```python
from build123d import *

# Parameters (mm, degrees)
CROQUIS1_R              = 2.6
CROQUIS1_R_2            = 3.5
CROQUIS1_R_3            = 1.75
CROQUIS1_R_4            = 11.25
CROQUIS1_R_5            = 2.5
CROQUIS1_W              = 7.5
CROQUIS1_H              = 3
SALIENTE_EXTRUIR1_DEPTH = 6


with BuildPart() as part:
    # Croquis1 → Saliente-Extruir1 (new body)
    with BuildSketch(Plane.XY):
        Polygon((-50, -104.5), (-50, 45.5), (-41, 54.5), (-41, 84.5), (-50, 89.696152423), (-50, 104.5), (50, 104.5), (50, 89.696152423), (41, 84.5), (41, 54.5), (50, 45.5), (50, -104.5), (27, -104.5), (21, -98.5), (-21, -98.5), (-27, -104.5), align=None)
        with Locations((-35, -94.5)):
            Circle(CROQUIS1_R, mode=Mode.SUBTRACT)
        with Locations((-35, -34.5)):
            Circle(CROQUIS1_R_2, mode=Mode.SUBTRACT)
        with Locations((35, -34.5)):
            Circle(CROQUIS1_R_2, mode=Mode.SUBTRACT)
        with Locations((35, -94.5)):
            Circle(CROQUIS1_R, mode=Mode.SUBTRACT)
        with Locations((-15.5, 13.5)):
            Circle(CROQUIS1_R_3, mode=Mode.SUBTRACT)
        with Locations((15.5, 13.5)):
            Circle(CROQUIS1_R_3, mode=Mode.SUBTRACT)
        with Locations((0, 29)):
            Circle(CROQUIS1_R_4, mode=Mode.SUBTRACT)
        with Locations((15.5, 44.5)):
            Circle(CROQUIS1_R_3, mode=Mode.SUBTRACT)
        with Locations((-15.5, 44.5)):
            Circle(CROQUIS1_R_3, mode=Mode.SUBTRACT)
        with Locations((0, 69.5)):
            Circle(CROQUIS1_R_5, mode=Mode.SUBTRACT)
        with Locations((0, 89.5)):
            Circle(CROQUIS1_R_5, mode=Mode.SUBTRACT)
        with Locations((0, 56)):
            Rectangle(CROQUIS1_W, CROQUIS1_H, mode=Mode.SUBTRACT)
        with Locations((0, 63)):
            Rectangle(CROQUIS1_W, CROQUIS1_H, mode=Mode.SUBTRACT)
    extrude(amount=SALIENTE_EXTRUIR1_DEPTH)


solid = part.part
```
Design review of the part built by this model. Coordinates are the model's own, in mm. A direction names the side the tool comes from. Give positions to 0.01 mm unless a question says otherwise; leave off trailing zeros. Write each loop counter-clockwise with the first axis right and the second up, starting at its lowest first coordinate (ties: lowest second). Pieces come first, ordered by that corner, then holes.
(1) Tool access review of faces 1 (the face through (50, 97, 3)), 2 (the face through (0, -98.5, 3)), 3 (the face through (0, 64.5, 3)), 4 (the face through (-45.437, 87.062, 2.958)), 5 (the face through (-50, -31, 3)): name each direction out of +Z, -Z, +X, -X, +Y, -Y from which nothing blocks a thin tool from reaching the whole face with its end or side.
Checked values:
face 1: +Z, -Z, +X, +Y, -Y
face 2: +Z, -Z, -Y
face 3: +Z, -Z
face 4: +Z, -Z, -X
face 5: +Z, -Z, -X, +Y, -Y
(2) Wall thickness on line 1 along Y through (x, z) = (15.5, 2.6); line 2 along Y through (x, z) = (35, 4.05); line 3 along Y through (x, z) = (-1, 0.9): over which ranges is each line inside the solid? List them lowest first.
Checked values:
line 1: y = -98.5 to 11.75, 15.25 to 42.75, 46.25 to 104.5
line 2: y = -104.5 to -97.1, -91.9 to -38, -31 to 104.5
line 3: y = -98.5 to 17.79, 40.21 to 54.5, 57.5 to 61.5, 64.5 to 67.21, 71.79 to 87.21, 91.79 to 104.5
(3) Add section C-C (x = 35). Give the boundary of the cut face in (y, z).
Checked values:
outline: (-104.5, 0) - (-97.1, 0) - (-97.1, 6) - (-104.5, 6) - close; (-91.9, 0) - (-38, 0) - (-38, 6) - (-91.9, 6) - close; (-31, 0) - (104.5, 0) - (104.5, 6) - (-31, 6) - close
(4) Add section B-B (y = 69.5). Give the boundary of the cut face in (x, z), and give its area (3 significant figures).
Checked values:
outline: (-41, 0) - (-2.5, 0) - (-2.5, 6) - (-41, 6) - close; (2.5, 0) - (41, 0) - (41, 6) - (2.5, 6) - close
area: 462 mm2
(5) Add section D-D (z = 4.1). Give the number of separate pieces and of enclosed holes in the cut face, and give its area (3 significant figures).
Checked values:
separate pieces: 1
enclosed holes: 13
area: 19,300 mm2
(6) Mouldability with a two-part tool opening along Y and no side actions: class faces 6 (the face through (-0.54, 67.06, 2.96)), 7 (the face through (50, -28, 3)), 8 (the face through (24, -101.5, 3)) as +Y half, -Y half, draft (parallel to the pull), parting line (faces both ways), or undercut.
Checked values:
face 6: undercut
face 7: draft
face 8: -Y half
(7) Clearance check with flat-ended pins moving along their axes: pin 1 Ø3 at (x, y) = (-15.5, 13.5) entering from -Z; pin 2 Ø2.5 at (y, z) = (56.5, 4) entering from -X; pin 3 Ø3 at (y, z) = (71, 3) entering from +X; pin 4 Ø3.5 at (y, z) = (55.5, 2.5) entering from +X. State where each tip first meets the part, or that it passes through.
Checked values:
pin 1: passes through
pin 2: stops at x = -41
pin 3: stops at x = 41
pin 4: stops at x = 41.75
(8) Add section A-A (y = -34.5). Give the boundary of the cut face in (x, z).
Checked values:
outline: (-50, 0) - (-38.5, 0) - (-38.5, 6) - (-50, 6) - close; (-31.5, 0) - (31.5, 0) - (31.5, 6) - (-31.5, 6) - close; (38.5, 0) - (50, 0) - (50, 6) - (38.5, 6) - close
